Check sheet for the modelled part. Datum: model origin and axes. Units: mm. Face numbers are marked on the shaded views. A direction names the side the tool comes from. Round coordinates to 2 decimals unless told otherwise and drop trailing zeros. Order: outer loops, then holes, each group sorted by start corner. A loop starts at its lowest first (then second) coordinate and runs counter-clockwise, first axis right, second up.
Q1. Cross-section at C-C on y = 38.5. Record the cut outline in (x, z).
Q2. Cross-section at A-A on y = 13.5. Record the cut outline in (x, z).
Q3. Mould release check, pull along Z, two halves, no side actions. Record for the marked faces 3, 4, 5 and 6: +Z half, -Z half, draft (parallel to the pull), parting line (faces both ways), or undercut.
Q4. Depth check by flat-ended pin: P1, Ø8.5, axis at x = -4.5, z = 3.5, coming from the -Y side; P2, Ø2, axis at y = 18, z = -5.5, coming from the -X side; P3, Ø1.4, axis at x = 0, z = -2, coming from the +Y side; P4, Ø7, axis at y = 22, z = 0, coming from the -X side (3 decimals). Enter the tip coordinate at first touch or a pass-through.
Q5. Cross-section at D-D on z = 0.5. Record the cut outline in (x, y) (3 decimals).
Q6. Cross-section at B-B on x = 7. Record the cut outline in (y, z).
Q7. Set-up check for the marked faces 1 and 2: record each of +Z, -Z, +X, -X, +Y, -Y from which the full face is reachable in a straight line by a thin tool's end or side.
Q8. Scan lines: probe 1 along Z at (x, y) = (-7.5, 61); probe 2 along Z at (x, y) = (2, 11); probe 3 along Y at (x, z) = (0, 9.75). Record each from-to range of solid material in increasing order.
from build123d import *

# Parameters (mm, degrees)
SKETCH1_W               = 35.56
SKETCH1_H               = 38.1
BOSS_EXTRUDE1_DEPTH     = 63.5
SKETCH3_W               = 35.56
SKETCH3_H               = 10.16
CUT_EXTRUDE1_DEPTH      = 38.1
SKETCH4_W               = 35.56
SKETCH4_H               = 17.145
CUT_EXTRUDE2_DEPTH      = 19.05
SKETCH5_W               = 17.145
SKETCH5_H               = 10.16
CUT_EXTRUDE3_DEPTH      = 47.158865887
CUT_EXTRUDE4_DEPTH      = 71.21848261
CUT_EXTRUDE4_DEPTH_BACK = 71.21848261
SKETCH6_R               = 1.125


with BuildPart() as part:
    # Sketch1 → Boss-Extrude1 (new body)
    with BuildSketch(Plane(origin=(0, 0, 0), x_dir=(1, 0, 0), z_dir=(0, 1, 0))):
        Rectangle(SKETCH1_W, SKETCH1_H)
    extrude(amount=BOSS_EXTRUDE1_DEPTH)

    # Sketch3 → Cut-Extrude1 (cut)
    with BuildSketch(Plane(origin=(0, 63.5, 0), x_dir=(1, 0, 0), z_dir=(0, 1, 0))):
        Rectangle(SKETCH3_W, SKETCH3_H)
    extrude(amount=-CUT_EXTRUDE1_DEPTH, mode=Mode.SUBTRACT)

    # Sketch4 → Cut-Extrude2 (cut)
    with BuildSketch(Plane.XZ):
        Rectangle(SKETCH4_W, SKETCH4_H)
    extrude(amount=-CUT_EXTRUDE2_DEPTH, mode=Mode.SUBTRACT)

    # Sketch5 → Cut-Extrude3 (cut, through all)
    with BuildSketch(Plane(origin=(0, 25.4, 0), x_dir=(1, 0, 0), z_dir=(0, 1, 0))):
        with Locations((-9.2075, 0)):
            Rectangle(SKETCH5_W, SKETCH5_H)
        with Locations((9.2075, 0)):
            Rectangle(SKETCH5_W, SKETCH5_H)
    extrude(amount=-CUT_EXTRUDE3_DEPTH, mode=Mode.SUBTRACT)

    # Sketch6 → Cut-Extrude4 (cut, two sides: drawn at the far end of the back side and taken through both)
    with BuildSketch(Plane.XY.offset(-5.08).offset(-CUT_EXTRUDE4_DEPTH_BACK)):
        with Locations((0, 29.845)):
            Circle(SKETCH6_R)
    extrude(amount=CUT_EXTRUDE4_DEPTH + CUT_EXTRUDE4_DEPTH_BACK, mode=Mode.SUBTRACT)


solid = part.part
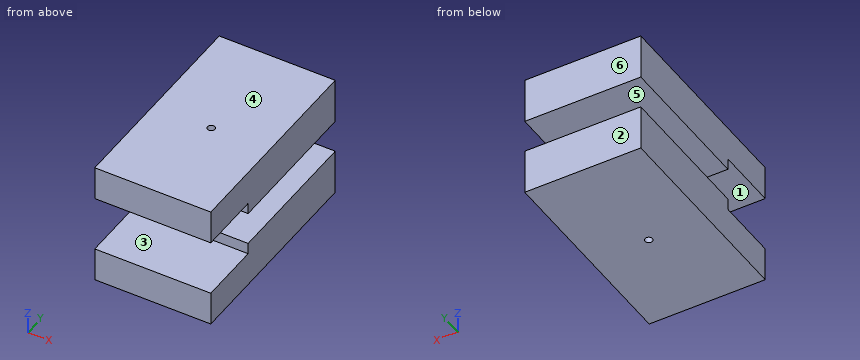
Results found:
1. outline: (-17.78, -19.05) - (17.78, -19.05) - (17.78, -5.08) - (-17.78, -5.08) - close; (-17.78, 5.08) - (17.78, 5.08) - (17.78, 19.05) - (-17.78, 19.05) - close
2. outline: (-17.78, -19.05) - (17.78, -19.05) - (17.78, -8.57) - (-17.78, -8.57) - close; (-17.78, 8.57) - (17.78, 8.57) - (17.78, 19.05) - (-17.78, 19.05) - close
3. face 3: undercut
3. face 4: +Z half
3. face 5: undercut
3. face 6: draft
4. P1: stops at y = 19.05
4. P2: passes through
4. P3: stops at y = 25.4
4. P4: stops at x = -0.635
5. outline: (-0.635, 19.05) - (0.635, 19.05) - (0.635, 25.4) - (-0.635, 25.4) - close
6. outline: (0, -19.05) - (63.5, -19.05) - (63.5, -5.08) - (19.05, -5.08) - (19.05, -8.57) - (0, -8.57) - close; (0, 8.57) - (19.05, 8.57) - (19.05, 5.08) - (63.5, 5.08) - (63.5, 19.05) - (0, 19.05) - close
7. face 1: +X, -X, -Y
7. face 2: +Z, -Z, +X, -X, +Y
8. probe 1: z = -19.05 to -5.08, 5.08 to 19.05
8. probe 2: z = -19.05 to -8.57, 8.57 to 19.05
8. probe 3: y = 0 to 28.72, 30.97 to 63.5
